Answer from the drawing. Dimensions are ordinates in mm from the lowest x, y and z of the part. A direction names the side the tool comes from. Round coordinates to 2 decimals unless told otherwise and drop trailing zeros. Loops run counter-clockwise (first coordinate to the right, second up) from the corner with the lowest first, then second, coordinate; pieces in that order, holes last. Notation, with made-up numbers: M -38.5,-21 L -11.5,-21 A16 ccw -11.5,7 Z; hole C -31.5,71 d8. An arc over 180 degrees is marked long. Answer as CSV lines item,"result".
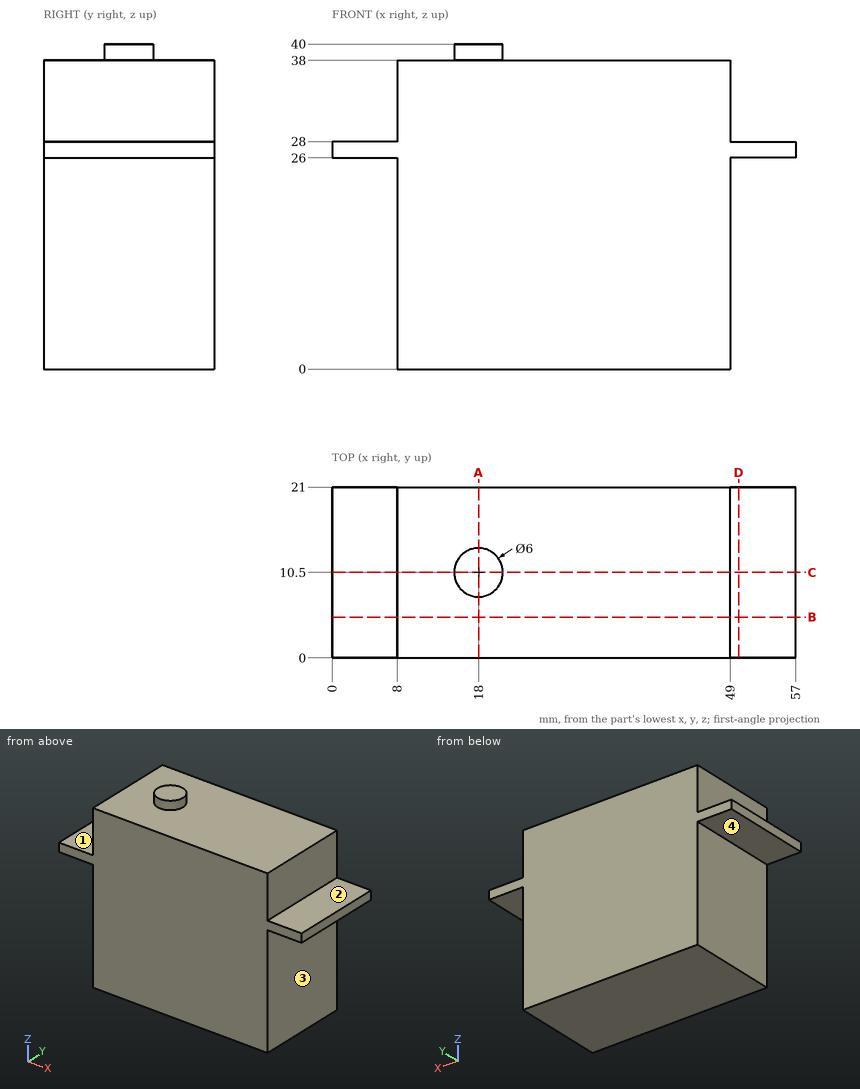
1) Find section C-C, the plane y = 10.5. Give the vertices of the cut face in (x, z), then the cut area to 3 significant figures.
Evaluation:
outline,"M 0,26 L 8,26 L 8,0 L 49,0 L 49,26 L 57,26 L 57,28 L 49,28 L 49,38 L 21,38 L 21,40 L 15,40 L 15,38 L 8,38 L 8,28 L 0,28 Z"
area,"1,600 mm^2"
2) Find section A-A, the plane x = 18. Give the vertices of the cut face in (y, z), then the cut area to 3 significant figures.
Evaluation:
outline,"M 0,0 L 21,0 L 21,38 L 13.5,38 L 13.5,40 L 7.5,40 L 7.5,38 L 0,38 Z"
area,"810 mm^2"
3) Each of these flat-tipped pins is pushed along its axis until it touches: P1, Ø5, axis at y = 10, z = 35, coming from the -X side; P2, Ø5, axis at y = 12.5, z = 35.5, coming from the +X side; P3, Ø1.5, axis at x = 6, y = 6, coming from the -Z side. Where does it stop, or does it pass through?
Evaluation:
P1,"stops at x = 8"
P2,"stops at x = 49"
P3,"stops at z = 26"
4) Find section D-D, the plane x = 50. Give the vertices of the cut face in (y, z), then the cut area to 3 significant figures.
Evaluation:
outline,"M 0,26 L 21,26 L 21,28 L 0,28 Z"
area,"42.0 mm^2"
5) Straight lines are drawn through the part: line 1 (X direction, y = 12.25, z = 30.5); line 2 (Z direction, x = 6, y = 8); line 3 (Z direction, x = 21, y = 19.25). For each, find the intervals that lie inside material, in ascending order.
Evaluation:
line 1,"x = 8 to 49"
line 2,"z = 26 to 28"
line 3,"z = 0 to 38"
6) A tool of negligible diameter and unlimited length cuts with its end or side. For the marked faces 1, 2, 3 and 4, from which of +Z, -Z, +X, -X, +Y, -Y can it reach the whole face along a straight path? Write none if from no direction.
Evaluation:
face 1,"+Z, -X, +Y, -Y"
face 2,"+Z, +X, +Y, -Y"
face 3,"-Z, +X, +Y, -Y"
face 4,"-Z, -X, +Y, -Y"
7) Find section B-B, the plane y = 5. Give the vertices of the cut face in (x, z).
Evaluation:
outline,"M 0,26 L 8,26 L 8,0 L 49,0 L 49,26 L 57,26 L 57,28 L 49,28 L 49,38 L 8,38 L 8,28 L 0,28 Z"
